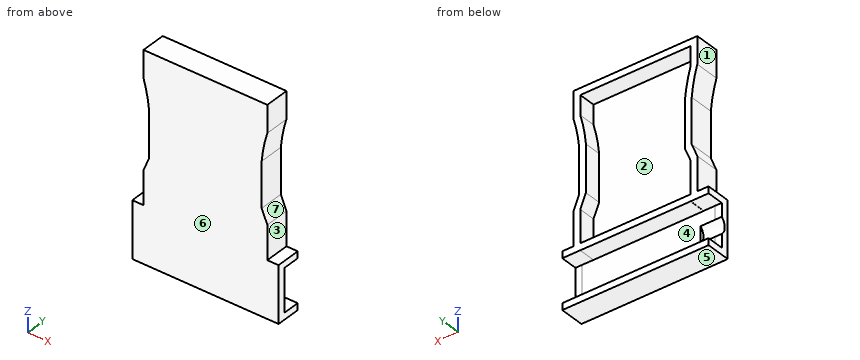
from build123d import *

# Parameters (mm, degrees)
BOSS_EXTRUDE1_DEPTH     = 18.415
CUT_EXTRUDE1_DEPTH      = 12.7
CUT_EXTRUDE2_DEPTH      = 116.078
CUT_EXTRUDE2_DEPTH_BACK = 116.078
SKETCH11_W              = 32.294856704
SKETCH11_H              = 12.721148442
SKETCH12_W              = 82.9732402
SKETCH12_H              = 5.08
BOSS_EXTRUDE3_DEPTH     = 12.7
SKETCH13_R              = 8.001
CUT_EXTRUDE3_DEPTH      = 16.002


with BuildPart() as part:
    # Sketch3 → Boss-Extrude1 (new body)
    with BuildSketch(Plane(origin=(0, 0, 0), x_dir=(1, 0, 0), z_dir=(0, 1, 0))):
        with BuildLine():
            Line((101.599873, 0), (110.066582, 0))
            Line((110.066582, 0), (110.066582, 42.333418))
            Line((110.066582, 42.333418), (55.033291, 42.333418))
            Line((55.033291, 42.333418), (8.4666328, 42.333418))
            Line((8.4666328, 42.333418), (0, 42.333418))
            Line((0, 42.333418), (0, 0))
            Line((0, 0), (8.4666328, 0))
            Line((8.4666328, 0), (8.4666328, -25.4))
            Line((8.4666328, -25.4), (12.6999492, -35.56))
            Line((12.6999492, -35.56), (12.6999492, -69.426582))
            add(Edge.make_bspline(
                [(12.6999492, -69.426582), (11.690404189, -80.766544706), (8.46666328, -91.44)],
                knots=[0, 0, 0, 0.504540069, 0.504540069, 0.504540069], degree=2))
            Line((8.46666328, -91.44), (8.46666328, -111.76))
            Line((8.46666328, -111.76), (101.599995682, -111.76))
            Line((101.599995682, -111.76), (101.599995682, -91.44))
            add(Edge.make_bspline(
                [(97.366709, -69.426582), (98.376270675, -80.766537876), (101.599995682, -91.44)],
                knots=[0, 0, 0, 0.504540407, 0.504540407, 0.504540407], degree=2))
            Line((97.366709, -69.426582), (97.366709, -35.56))
            Line((97.366709, -35.56), (101.599873, -25.4))
            Line((101.599873, -25.4), (101.599873, 0))
        make_face()
    extrude(amount=BOSS_EXTRUDE1_DEPTH)

    # Sketch7 → Cut-Extrude1 (cut)
    with BuildSketch(Plane(origin=(0, 18.415, 0), x_dir=(1, 0, 0), z_dir=(0, 1, 0))):
        with BuildLine():
            Line((104.986582, 5.08), (104.986582, 37.253418))
            Line((104.986582, 37.253418), (5.08, 37.253418))
            Line((5.08, 37.253418), (5.08, 5.08))
            Line((5.08, 5.08), (13.5466328, 5.08))
            Line((13.5466328, 5.08), (13.5466328, -24.384003751))
            Line((13.5466328, -24.384003751), (17.7799492, -34.544003751))
            Line((17.7799492, -34.544003751), (17.7799492, -69.649806794))
            add(Edge.make_bspline(
                [(13.54666328, -92.18157962), (15.696718758, -84.885689198), (17.107633166, -77.368389863), (17.7799492, -69.649806794)],
                knots=[0, 0, 0, 0, 1, 1, 1, 1], degree=3))
            Line((13.54666328, -92.18157962), (13.54666328, -106.68))
            Line((13.54666328, -106.68), (96.519995682, -106.68))
            Line((96.519995682, -106.68), (96.519995682, -92.1815758))
            add(Edge.make_bspline(
                [(92.286709, -69.649810631), (92.959036165, -77.368387225), (94.369950858, -84.885683715), (96.519995682, -92.1815758)],
                knots=[0, 0, 0, 0, 1, 1, 1, 1], degree=3))
            Line((92.286709, -69.649810631), (92.286709, -34.544037514))
            Line((92.286709, -34.544037514), (96.519873, -24.384037514))
            Line((96.519873, -24.384037514), (96.519873, 5.08))
            Line((96.519873, 5.08), (104.986582, 5.08))
        make_face()
    extrude(amount=-CUT_EXTRUDE1_DEPTH, mode=Mode.SUBTRACT)

    # Sketch11 → Cut-Extrude2 (cut, two sides: drawn at the far end of the back side and taken through both)
    with BuildSketch(Plane(origin=(105.08, 0, 0), x_dir=(0, 0, -1), z_dir=(1, 0, 0)).offset(-CUT_EXTRUDE2_DEPTH_BACK)):
        with Locations((21.166087112, 12.087958035)):
            Rectangle(SKETCH11_W, SKETCH11_H)
    extrude(amount=CUT_EXTRUDE2_DEPTH + CUT_EXTRUDE2_DEPTH_BACK, mode=Mode.SUBTRACT)

    # Sketch12 → Boss-Extrude3 (add)
    with BuildSketch(Plane(origin=(0, 18.415, 0), x_dir=(1, 0, 0), z_dir=(0, 1, 0))):
        with Locations((55.0332529, 2.54)):
            Rectangle(SKETCH12_W, SKETCH12_H)
    extrude(amount=-BOSS_EXTRUDE3_DEPTH)

    # Sketch13 → Cut-Extrude3 (cut)
    with BuildSketch(Plane.ZY):
        with Locations((-21.166398056, 10.864691907)):
            Circle(SKETCH13_R)
    extrude(amount=-CUT_EXTRUDE3_DEPTH, mode=Mode.SUBTRACT)


solid = part.part
The listing builds one solid part. Answer for the finished solid, in the listing's coordinates (mm). Face numbers are marked on the shaded views. A direction names the side the tool comes from. Round coordinates to 2 decimals unless told otherwise and drop trailing zeros. Order: outer loops, then holes, each group sorted by start corner. A loop starts at its lowest first (then second) coordinate and runs counter-clockwise, first axis right, second up. Notation, with made-up numbers: M 71.5,25 L 101.5,25 A24 ccw 101.5,60 Z; hole C -27,63.25 d5. An arc over 180 degrees is marked long. Answer in a Markdown table with one row per item. Add a question column.
1) The part is cut by section C-C on y = 14.75. Count the separate pieces of the cut face and the enclosed holes in it, plus the area to 3 significant figures.
2) Flat-ended cylindrical pins translate along their axes: pin 1 Ø2 at (y, z) = (15.5, 27.5) entering from -X; pin 2 Ø5 at (x, z) = (28, 77) entering from +Y (3 decimals); pin 3 Ø5.5 at (y, z) = (7.5, 101.5) entering from +X; pin 4 Ø8 at (x, z) = (36.5, 88.5) entering from -Y. Find the tip coordinate at first contact, or state that the pin passes through.
3) The part is cut by section D-D on z = -31.5. Determine the outline of the cut face in (x, y) (3 decimals).
4) Consider line 1 along Z through (x, y) = (76, 9); line 2 along X through (y, z) = (16.75, 103); line 3 along X through (y, z) = (12.5, 62). Determine where each line is inside the solid, lowest interval first. Write a range as from..to.
5) The part is cut by section B-B on x = 85.5. Determine the outline of the cut face in (y, z) (3 decimals), plus the area to 3 significant figures.
6) The part is cut by section A-A on z = 48.5. Determine the outline of the cut face in (x, y) (3 decimals), plus the area to 3 significant figures.
7) Determine the mould class of the marked faces 5, 6 and 7 for opening direction Z: pulls with the +Z half, pulls with the -Z half, needs draft (parallel to the pull), parting line crosses it, or undercut.
8) Which of the six approach directions +Z, -Z, +X, -X, +Y, -Y give full straight-line access (tool end or side, diameter ignored) to the marked faces 1, 2, 3 and 4?
Findings below:
| question | item | result |
|---|---|---|
| 1 | separate pieces | 2 |
| 1 | enclosed holes | 1 |
| 1 | area | 2,680 mm² |
| 2 | pin 1 | stops at x = 8.92 |
| 2 | pin 2 | stops at y = 5.715 |
| 2 | pin 3 | stops at x = 101.6 |
| 2 | pin 4 | stops at y = 0 |
| 3 | outline | M 0,0 L 110.067,0 L 110.067,5.727 L 104.987,5.727 L 104.987,5.715 L 5.08,5.715 L 5.08,5.727 L 0,5.727 Z |
| 4 | line 1 | z = -42.33..-37.31, -5.08..0, 106.68..111.76 |
| 4 | line 2 | x = 8.47..13.55, 96.52..101.6 |
| 4 | line 3 | x = 12.7..17.78, 92.29..97.37 |
| 5 | outline | M 0,-42.333 L 18.415,-42.333 L 18.415,-37.314 L 5.727,-37.314 L 5.727,-37.253 L 5.715,-37.253 L 5.715,-5.08 L 18.415,-5.08 L 18.415,0 L 5.715,0 L 5.715,106.68 L 18.415,106.68 L 18.415,111.76 L 0,111.76 Z |
| 5 | area | 1,070 mm² |
| 6 | outline | M 12.7,0 L 97.367,0 L 97.367,18.415 L 92.287,18.415 L 92.287,5.715 L 17.78,5.715 L 17.78,18.415 L 12.7,18.415 Z |
| 6 | area | 613 mm² |
| 7 | face 5 | pulls with the -Z half |
| 7 | face 6 | needs draft |
| 7 | face 7 | undercut |
| 8 | face 1 | +Z, -X, +Y, -Y |
| 8 | face 2 | +Y |
| 8 | face 3 | +Z, +X, +Y, -Y |
| 8 | face 4 | +X, -X, +Y |
